from build123d import *

# Parameters (mm, degrees)
SKETCH_R        = 2.175
PAD_DEPTH       = 7
SKETCH001_R     = 1.4
PAD001_DEPTH    = 1.4
SKETCH002_R     = 1
POCKET_DEPTH    = 8.401
CHAMFER_SIZE    = 0.3
CHAMFER001_SIZE = 0.3
FILLET_R        = 0.1


with BuildPart() as part:
    # Sketch → Pad (new body)
    with BuildSketch(Plane.XY):
        Circle(SKETCH_R)
    extrude(amount=PAD_DEPTH)

    # Sketch001 (on Face2 of Pad) → Pad001 (join)
    with BuildSketch(Plane(origin=(0, 0, 0), x_dir=(1, 0, 0), z_dir=(0, 0, -1))):
        Circle(SKETCH001_R)
    extrude(amount=PAD001_DEPTH)

    # Sketch002 (on Face5 of Pad001) → Pocket (cut, through all)
    with BuildSketch(Plane(origin=(0, 0, -1.4), x_dir=(1, 0, 0), z_dir=(0, 0, -1))):
        Circle(SKETCH002_R)
    extrude(amount=-POCKET_DEPTH, mode=Mode.SUBTRACT)

    # Chamfer
    chamfer_edges = [part.edges().sort_by_distance(p)[0] for p in [
        (-1.4, 0, -1.4),
    ]]
    chamfer(chamfer_edges, length=CHAMFER_SIZE)

    # Chamfer001
    chamfer001_edges = [part.edges().sort_by_distance(p)[0] for p in [
        (-2.175, 0, 7),
    ]]
    chamfer(chamfer001_edges, length=CHAMFER001_SIZE)

    # Fillet
    fillet_edges = [part.edges().sort_by_distance(p)[0] for p in [
        (-2.175, 0, 0),
    ]]
    fillet(fillet_edges, radius=FILLET_R)


solid = part.part
Read the model definition and answer for the solid it produces. Units are mm, in the model's axes. Coordinates: 2 decimals unless noted, no trailing zeros. Loops run counter-clockwise (first coordinate to the right, second up) from the corner with the lowest first, then second, coordinate; pieces in that order, holes last. Notation, with made-up numbers: (35.25, 43.25) -> (58.25, 43.25) arc R15 cw to (58.25, 71.25) -> close; hole circle Ø8 at (28.5, 9). An arc over 180 degrees is marked (long way). Answer in a Markdown table with one row per item.
Item 1: For a pull along X with two mould halves and no side action, classify faces 1 (the cylindrical face through (-1.4, -0.06, -0.54)), 2 (the flat face through (1, -1, 7)), 3 (the cylindrical face through (0, 1, 3)) as released by +X, released by -X, zero draft, split by the parting line, or undercut.
Returned:
| item | result |
|---|---|
| face 1 | split by the parting line |
| face 2 | zero draft |
| face 3 | undercut |
Item 2: A cutting plane is placed at C-C on z = 4.5. Determine the outline of the cut face in (x, y) (3 decimals), plus the area to 3 significant figures.
Returned:
| item | result |
|---|---|
| outline | circle Ø4.35 at (0, 0); hole circle Ø2 at (0, 0) |
| area | 11.7 mm^2 |
Item 3: A cutting plane is placed at A-A on y = 0. Determine the outline of the cut face in (x, z) (3 decimals), plus the area to 3 significant figures.
Returned:
| item | result |
|---|---|
| outline | (-2.175, 0.1) arc R0.1 ccw to (-2.075, 0) -> (-1.4, 0) -> (-1.4, -1.1) -> (-1.1, -1.4) -> (-1, -1.4) -> (-1, 7) -> (-1.875, 7) -> (-2.175, 6.7) -> close; (1, -1.4) -> (1.1, -1.4) -> (1.4, -1.1) -> (1.4, 0) -> (2.075, 0) arc R0.1 ccw to (2.175, 0.1) -> (2.175, 6.7) -> (1.875, 7) -> (1, 7) -> close |
| area | 17.4 mm^2 |
Item 4: Straight lines are drawn through the part: line 1 along Y through (x, z) = (0, 1.25) (3 decimals); line 2 along Y through (x, z) = (0.65, 1.25); line 3 along Z through (x, y) = (-0.95, -1.15). For each, find the intervals that lie inside material, in ascending order. Write a range as [from, to].
Returned:
| item | result |
|---|---|
| line 1 | y = [-2.175, -1], [1, 2.175] |
| line 2 | y = [-2.08, -0.76], [0.76, 2.08] |
| line 3 | z = [0, 7] |
Item 5: This flat-tipped pin is pushed along its axis until it touches: P1, Ø1, axis at y = 1.5, z = 4.5, coming from the +X side. Where does it stop, or does it pass through?
Returned:
| item | result |
|---|---|
| P1 | stops at x = 1.93 |
